Source: three-view drawing plus pictorial views. Frame: mm from the lowest corner of the part. A direction names the side the tool comes from. Give positions to 0.01 mm unless a question says otherwise; leave off trailing zeros. Order: outer loops, then holes, each group sorted by start corner. A loop starts at its lowest first (then second) coordinate and runs counter-clockwise, first axis right, second up. Notation, with made-up numbers: (2.25, 4.5) - (49.25, 4.5) arc R14 ccw to (49.25, 20.5) - close; hole circle Ø1 at (82.5, 66). An arc over 180 degrees is marked (long way). Use one line per item in the form item = value.
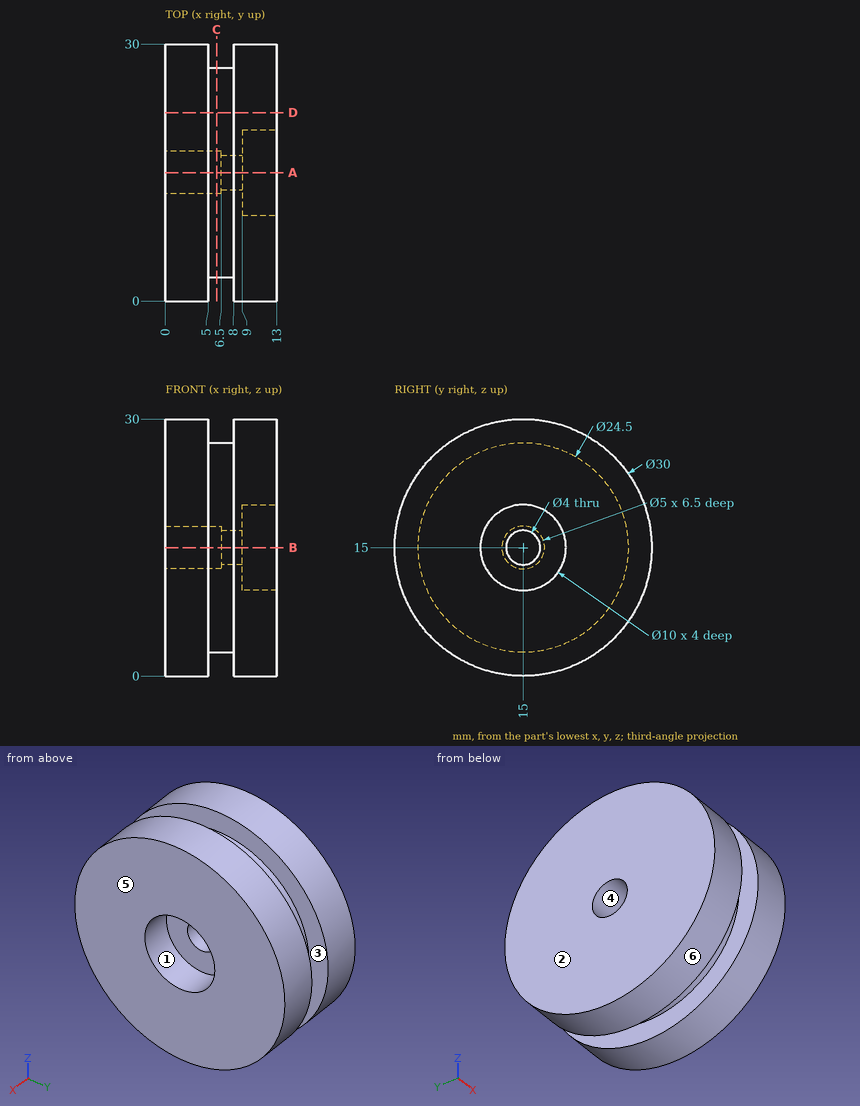
(1) Cut plane C-C on x = 6. Output: boundary loops of the cut face in (y, z), plus the area to 3 significant figures.
Computed values:
outline = circle Ø24.5 at (15, 15); hole circle Ø5 at (15, 15)
area = 452 mm²
(2) Pull-direction query (Y, two-part tool) for the marked faces 4, 5 and 6; classes: released by +Y, released by -Y, zero draft, split by the parting line, or undercut.
Computed values:
face_4 = undercut
face_5 = zero draft
face_6 = split by the parting line
(3) Ray query, line 1 along Y through (x, z) = (4.5, 15); line 2 along Z through (x, y) = (9.5, 15.25); line 3 along Y through (x, z) = (11.9, 15). Return the intervals inside material, ascending.
Computed values:
line_1 = 0 to 12.5, 17.5 to 30
line_2 = 0 to 10.01, 19.99 to 30
line_3 = 0 to 10, 20 to 30
(4) Cut plane A-A on y = 15. Output: boundary loops of the cut face in (x, z).
Computed values:
outline = (0, 0) - (5, 0) - (5, 2.75) - (8, 2.75) - (8, 0) - (13, 0) - (13, 10) - (9, 10) - (9, 13) - (6.5, 13) - (6.5, 12.5) - (0, 12.5) - close; (0, 17.5) - (6.5, 17.5) - (6.5, 17) - (9, 17) - (9, 20) - (13, 20) - (13, 30) - (8, 30) - (8, 27.25) - (5, 27.25) - (5, 30) - (0, 30) - close
(5) Contact query for flat-ended pins moving along their axis: pin 1 Ø4.5 at (y, z) = (15, 15) entering from -X; pin 2 Ø2.5 at (y, z) = (15, 15.5) entering from -X (1 decimal); pin 3 Ø4 at (x, z) = (4.5, 13.5) entering from -Y; pin 4 Ø1.5 at (x, y) = (6, 24) entering from -Z. Output: stop coordinate, or through.
Computed values:
pin_1 = 6.5
pin_2 = through
pin_3 = 0
pin_4 = 5.94
(6) Cut plane D-D on y = 22. Output: boundary loops of the cut face in (x, z), plus the area to 3 significant figures.
Computed values:
outline = (0, 1.73) - (5, 1.73) - (5, 4.95) - (8, 4.95) - (8, 1.73) - (13, 1.73) - (13, 28.27) - (8, 28.27) - (8, 25.05) - (5, 25.05) - (5, 28.27) - (0, 28.27) - close
area = 326 mm²
(7) Reachability of the marked faces 1, 2 and 3 from +Z, -Z, +X, -X, +Y, -Y: full face, straight path, thin tool, end or side. Return the list, or none.
Computed values:
face_1 = +X
face_2 = +Z, -Z, -X, +Y, -Y
face_3 = none
